Check sheet for the modelled part. Datum: model origin and axes. Units: mm. A direction names the side the tool comes from. Round coordinates to 2 decimals unless told otherwise and drop trailing zeros. Order: outer loops, then holes, each group sorted by start corner. A loop starts at its lowest first (then second) coordinate and runs counter-clockwise, first axis right, second up.
from build123d import *

# Parameters (mm, degrees)
F0_W     = 100
F0_H     = 60
F0_W_2   = 90
F0_H_2   = 50
F0_W_3   = 80
F0_H_3   = 40
F1_DEPTH = 8
F2_DEPTH = 5
F4_DEPTH = 10
F5_R     = 5
F6_R     = 7.243557
F7_DEPTH = 10
F8_R     = 5


with BuildPart() as f1:
    # F0 (on Top) → F1 (new body)
    with BuildSketch(Plane.XY):
        with Locations((9.720059, 5.494498)):
            Rectangle(F0_W, F0_H)
        with Locations((9.720059, 5.494498)):
            Rectangle(F0_W_2, F0_H_2, mode=Mode.SUBTRACT)
        with Locations((9.720059, 5.494498)):
            Rectangle(F0_W_3, F0_H_3)
    extrude(amount=F1_DEPTH)

    # F0 (on Top) → F2 (join)
    with BuildSketch(Plane.XY):
        with Locations((9.720059, 5.494498)):
            Rectangle(F0_W_2, F0_H_2)
        with Locations((9.720059, 5.494498)):
            Rectangle(F0_W_3, F0_H_3, mode=Mode.SUBTRACT)
    extrude(amount=F2_DEPTH)

    # F3 (on face) → F4 (join)
    with BuildSketch(Plane.XY.offset(8)):
        Polygon((9.720059, 21.794148), (-25.105188, 5.494498), (9.720059, -11.379591), (44.720059, 6.427957), align=None)
    extrude(amount=F4_DEPTH)

    # F5
    f5_edges = [f1.edges().sort_by_distance(p)[0] for p in [
        (54.720059, -19.505502, 6.5),
        (-35.279941, -19.505502, 6.5),
        (-35.279941, 30.494498, 6.5),
        (54.720059, 30.494498, 6.5),
        (-30.279941, 25.494498, 6.5),
        (-30.279941, -14.505502, 6.5),
        (49.720059, -14.505502, 6.5),
        (49.720059, 25.494498, 6.5),
        (44.720059, 6.427957, 13),
        (9.720059, 21.794148, 13),
        (9.720059, -11.379591, 13),
        (-25.105188, 5.494498, 13),
    ]]
    fillet(f5_edges, radius=F5_R)

    # F6 (on face) → F7 (join)
    with BuildSketch(Plane.XY.offset(18)):
        with Locations((9.861113, 5.972222)):
            Circle(F6_R)
    extrude(amount=F7_DEPTH)

    # F8
    f8_edges = [f1.edges().sort_by_distance(p)[0] for p in [
        (59.720059, -24.505502, 4),
        (-40.279941, -24.505502, 4),
        (-40.279941, 35.494498, 4),
        (59.720059, 35.494498, 4),
    ]]
    fillet(f8_edges, radius=F8_R)


solid = f1.part
1) Set-up check for faces 5 (the face through (48.294, 23.991, 6.521)), 6 (the face through (9, -24.506, 4)): record each of +Z, -Z, +X, -X, +Y, -Y from which the full face is reachable in a straight line by a thin tool's end or side.
2) Gauge pin test, flat ends, axial feed: pin 1 (12 mm diameter, centred on x = 21.5, z = 16, fed in from -Y); pin 2 (5 mm diameter, centred on y = 17, z = 18.5, fed in from +X); pin 3 (5 mm diameter, centred on x = -18, y = 28.5, fed in from +Z); pin 4 (6 mm diameter, centred on x = -22, z = 14.5, fed in from +Y). Record the tip position at first contact, or that the pin passes through.
3) Draft check along X on faces 1 (the face through (2.625, 6.291, 22.93)), 2 (the face through (-33.776, -18.08, 6.521)), 3 (the face through (58.217, -23.08, 4.056)), 4 (the face through (-33.776, 29.069, 6.521)). Enter one of: pulls with the +X half, pulls with the -X half, needs draft (parallel to the pull), parting line crosses it, or undercut.
4) Sectioned sample at C-C on y = 29.5. Record the cut outline in (x, z).
5) Sectioned sample at B-B on x = 42. Record the cut outline in (y, z), and give its area (3 significant figures).
6) Sectioned sample at A-A on z = 6. Record the cut outline in (x, y), and give its area (3 significant figures).
7) Scan lines: line 1 (Y direction, x = 17, z = 6); line 2 (X direction, y = -11.5, z = 6); line 3 (Z direction, x = 45, y = 33). Record each from-to range of solid material in increasing order.
8) Sectioned sample at D-D on z = 13.25. Record the cut outline in (x, y), and give its area (3 significant figures).
Values found:
1. face 5: +Z
1. face 6: +Z, -Z, +X, -X, -Y
2. pin 1: stops at y = -8.44
2. pin 2: stops at x = 26.22
2. pin 3: stops at z = 8
2. pin 4: passes through
3. face 1: parting line crosses it
3. face 2: undercut
3. face 3: pulls with the +X half
3. face 4: undercut
4. outline: (-40.28, 0) - (59.72, 0) - (59.72, 8) - (52.71, 8) - (52.71, 5) - (-33.27, 5) - (-33.27, 8) - (-40.28, 8) - close
5. outline: (-24.51, 0) - (35.49, 0) - (35.49, 8) - (30.49, 8) - (30.49, 5) - (25.49, 5) - (25.49, 8) - (-14.51, 8) - (-14.51, 5) - (-19.51, 5) - (-19.51, 8) - (-24.51, 8) - close
5. area: 450 mm2
6. outline: (-40.28, -19.51) arc R5 ccw to (-35.28, -24.51) - (54.72, -24.51) arc R5 ccw to (59.72, -19.51) - (59.72, 30.49) arc R5 ccw to (54.72, 35.49) - (-35.28, 35.49) arc R5 ccw to (-40.28, 30.49) - close; (-30.28, -9.51) arc R5 ccw to (-25.28, -14.51) - (44.72, -14.51) arc R5 ccw to (49.72, -9.51) - (49.72, 20.49) arc R5 ccw to (44.72, 25.49) - (-25.28, 25.49) arc R5 ccw to (-30.28, 20.49) - close; hole (-35.28, -14.51) arc R5 ccw to (-30.28, -19.51) - (49.72, -19.51) arc R5 ccw to (54.72, -14.51) - (54.72, 25.49) arc R5 ccw to (49.72, 30.49) - (-30.28, 30.49) arc R5 ccw to (-35.28, 25.49) - close
6. area: 4,680 mm2
7. line 1: y = -24.51 to -19.51, -14.51 to 25.49, 30.49 to 35.49
7. line 2: x = -40.28 to -35.28, -29.86 to 49.31, 54.72 to 59.72
7. line 3: z = 0 to 8
8. outline: (-15.66, 0.92) - (7.49, -10.3) arc R5 ccw to (11.93, -10.25) - (35.31, 1.64) arc R5 ccw to (35.05, 10.67) - (11.8, 20.88) arc R5 ccw to (7.67, 20.83) - (-15.6, 9.94) arc R5 ccw to start
8. area: 1,110 mm2
